Read the model definition and answer for the solid it produces. Units are mm, in the model's axes. Face numbers are marked on the shaded views. Round coordinates to 2 decimals unless told otherwise and drop trailing zeros. Order: outer loops, then holes, each group sorted by start corner. A loop starts at its lowest first (then second) coordinate and runs counter-clockwise, first axis right, second up. Notation, with made-up numbers: (19.25, 88.25) -> (49.25, 88.25) arc R27 ccw to (49.25, 104.25) -> close; hole circle Ø6 at (89.5, 20.5). An arc over 180 degrees is marked (long way). Answer as a JSON object with one key per item and string values. Group by question number.
Item 1: Consider probe 1 along X at (y, z) = (0.6, -0.5); probe 2 along X at (y, z) = (0.05, 0); probe 3 along X at (y, z) = (1.65, 1.25). Determine where each line is inside the solid, lowest interval first. Write a range as from..to.
Item 2: Section C-C, the plane y = 0.7 is taken. Write down the section's boundary in (x, z), plus the area to 3 significant figures.
Item 3: Given P1, Ø1.5, axis at y = 2, z = 3.5, coming from the +X side; P2, Ø2, axis at x = 2, z = 0, coming from the +Y side; P3, Ø3, axis at x = -1.5, z = -2, coming from the -Y side, each flat-ended and moving along its own axis, determine where each tip first touches the part or whether it passes through.
Item 4: The mould has two halves that part along X. Classify the marked faces 1, 2 and 3: pulls with the +X half, pulls with the -X half, needs draft (parallel to the pull), parting line crosses it, or undercut.
Item 5: Section D-D, the plane y = 1.85 is taken. Write down the section's boundary in (x, z), plus the area to 3 significant figures.
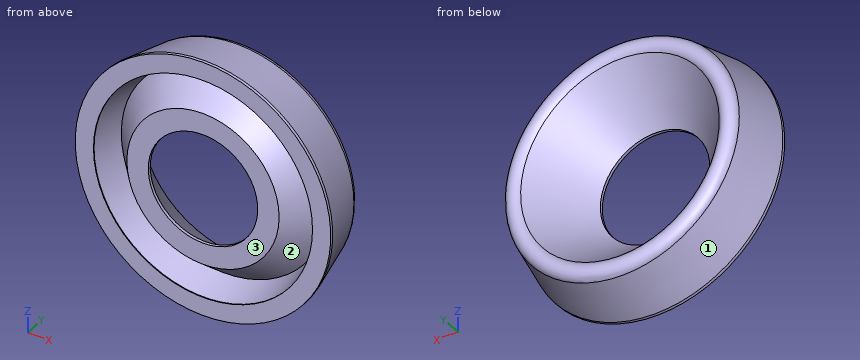
from build123d import *


# Read off the part's stored shape, not the designer's step: Shell2
with BuildPart() as part:
    # Sketch1 → Revolve1 (revolve)
    with BuildSketch(Plane.XY, mode=Mode.PRIVATE) as revolve1_sk:
        with BuildLine():
            Line((-5.55625, 0), (-5.55625, 0.127))
            Line((-5.55625, 0.127), (-5.070967234, 2.25500545))
            ThreePointArc((-5.070967234, 2.25500545), (-4.751339811, 2.57873382), (-4.319197328, 2.43655569))
            Line((-4.319197328, 2.43655569), (-2.38125, 0.127))
            Line((-2.38125, 0.127), (-2.38125, 0))
            Line((-2.38125, 0), (-5.55625, 0))
        make_face()
    revolve(revolve1_sk.sketch.rotate(Axis((0, 0, 0), (0, 1, 0)), 270), axis=Axis((0, 0, 0), (0, 1, 0)))

    # Shell2 outline → Shell2 (revolve, cut)
    with BuildSketch(Plane.XY):
        Polygon((4.459036573, 1.368353826), (3.310851383, 0), (4.7625, 0), (4.7625, 0.03764136), align=None)
    revolve(axis=Axis((0, 0, 0), (0, 1, 0)), mode=Mode.SUBTRACT)


solid = part.part
Values found:
{
 "1": {"probe 1": "-5.43..-4.61, -3.78..-2.73, 2.73..3.78, 4.61..5.43", "probe 2": "-5.56..-4.76, -3.35..-2.38, 2.38..3.35, 4.76..5.56", "probe 3": "-5.06..-3.44, 3.44..5.06"},
 "2": {"outline": "circle Ø10.85 at (0, 0); circle Ø7.8 at (0, 0); hole circle Ø9.22 at (0, 0); hole circle Ø5.72 at (0, 0)", "area": "47.7 mm2"},
 "3": {"P1": "x = 4.37", "P2": "y = 0.86", "P3": "y = 0"},
 "4": {"face 1": "parting line crosses it", "face 2": "undercut", "face 3": "needs draft"},
 "5": {"outline": "circle Ø10.33 at (0, 0); hole circle Ø7.65 at (0, 0)", "area": "37.7 mm2"}
}
